from build123d import *

# Parameters (mm, degrees)
SKETCH1_R           = 3.3
BOSS_EXTRUDE1_DEPTH = 4.7625
FILLET1_R           = 0.254


with BuildPart() as part:
    # Sketch1 → Boss-Extrude1 (new body)
    with BuildSketch(Plane(origin=(0, 0, 0), x_dir=(1, 0, 0), z_dir=(0, 1, 0))):
        with BuildLine():
            Line((17.670610129, -24.03336424), (-6.055469212, -11.163390731))
            ThreePointArc((-6.055469212, -11.163390731), (10.379538335, -7.318140744), (8.480594992, 9.453544763))
            Line((8.480594992, 9.453544763), (28.572658281, -8.570662619))
            ThreePointArc((28.572658281, -8.570662619), (29.996865789, -21.149426749), (17.670610129, -24.03336424))
        make_face()
        with Locations(Location((22.212212038, -15.660821191, 0), (0, 0, 90))):
            Circle(SKETCH1_R, mode=Mode.SUBTRACT)
    extrude(amount=BOSS_EXTRUDE1_DEPTH)

    # Fillet1
    fillet1_edges = [part.edges().sort_by_distance(p)[0] for p in [
        (-6.055469212, 2.38125, 11.163390731),
        (8.480594992, 2.38125, -9.453544763),
    ]]
    fillet(fillet1_edges, radius=FILLET1_R)


solid = part.part
Source: CAD feature listing. Evaluate the final solid. Frame: model axes, mm. Coordinates: 2 decimals unless noted, no trailing zeros. Order: outer loops, then holes, each group sorted by start corner. A loop starts at its lowest first (then second) coordinate and runs counter-clockwise, first axis right, second up.
Item 1: Pull-direction query (Z, two-part tool) for faces 1 (the face through (18, 4.762, 12)), 2 (the face through (10.258, 2.348, 7.488)), 3 (the face through (30.1, 2.3, 21)); classes: pulls with the +Z half, pulls with the -Z half, needs draft (parallel to the pull), parting line crosses it, or undercut.
Output values:
face 1: needs draft
face 2: undercut
face 3: parting line crosses it
Item 2: Cut plane C-C (y = 3.9). Return loops of the section in (x, z) (3 decimals), plus the area to 3 significant figures.
Output values:
outline: (-2.898, 12.876) arc R0.254 ccw to (-2.722, 12.405) arc R12.7 cw to (10.769, -6.731) arc R0.254 ccw to (11.154, -7.055) - (28.573, 8.571) arc R9.525 ccw to (17.671, 24.033) - close; hole circle Ø6.6 at (22.212, 15.661)
area: 462 mm2
Item 3: Cut plane B-B (z = 13.5). Return loops of the section in (x, y).
Output values:
outline: (-1.75, 0) - (19.72, 0) - (19.72, 4.76) - (-1.75, 4.76) - close; (24.71, 0) - (31.49, 0) - (31.49, 4.76) - (24.71, 4.76) - close
Item 4: Cut plane A-A (x = 21). Return loops of the section in (y, z), plus the area to 3 significant figures.
Output values:
outline: (0, 1.78) - (4.76, 1.78) - (4.76, 12.59) - (0, 12.59) - close; (0, 18.73) - (4.76, 18.73) - (4.76, 25.11) - (0, 25.11) - close
area: 81.9 mm2
Item 5: Cut plane D-D (z = 1). Return loops of the section in (x, y).
Output values:
outline: (12.66, 0) - (20.13, 0) - (20.13, 4.76) - (12.66, 4.76) - close
Item 6: First-contact query: P1, Ø1, axis at y = 1.5, z = -2.5, coming from the -X side. Flat tip, straight axial feed; report the tip coordinate or a pass-through.
Output values:
P1: stops at x = 12.34
Item 7: Material intervals for line 1 (Z direction, x = 20, y = 0.35); line 2 (X direction, y = 2.75, z = 5.5); line 3 (Z direction, x = 10.5, y = 3.05), sorted ascending.
Output values:
line 1: z = 0.88 to 13.21, 18.11 to 24.93
line 2: x = 11.45 to 25.15
line 3: z = 7.14 to 20.14
